For this review, take the finished solid that the model builds, in its own axes (mm). Round coordinates to 2 decimals unless told otherwise and drop trailing zeros. Write each loop counter-clockwise with the first axis right and the second up, starting at its lowest first coordinate (ties: lowest second). Pieces come first, ordered by that corner, then holes.
Autodesk Inventor part; units mm, degrees
ref_plane "YZ Plane" through (0, 0, 0) normal (1, 0, 0) x (0, 1, 0)
ref_plane "XZ Plane" through (0, 0, 0) normal (0, 1, 0) x (-1, 0, 0)
ref_plane "XY Plane" through (0, 0, 0) normal (0, 0, 1) x (1, 0, 0)
sketch "Sketch1" plane through (0, 0, 0) normal (0, 0, 1) x (1, 0, 0)
  circle A0 centre (0, 0) radius 35
  dimension "d0" = 70
extrude "Plate1" add sketch "Sketch1" along normal blind 2
sketch "Sketch2" plane through (0, 0, 0) normal (0, 0, 1) x (1, 0, 0)
  point P0 (0, 0)
  point P1 (28, 0)
  dimension "d2" = 28
hole "Hole1" at (28, 0, 0) direction (0, 0, 1) diameter 6 end through all
pattern_circular "Circular Pattern1" count 3 over 360 about axis through (0, 0, -10) along (0, 0, 1) of "Hole1"
sketch "Sketch3" plane through (0, 0, 2) normal (0, 0, 1) x (1, 0, 0)
  circle A0 centre (0, 0) radius 16.05
  dimension "d13" = 32.1
extrude "Extrusion1" cut sketch "Sketch3" against normal through all
equation "\"d0\" = Внешний_диам_фланца"
equation "\"d8\" = Thickness"
equation "\"d1\" = Thickness"
equation "\"BendRadius\" = Thickness"
equation "\"BendReliefWidth\" = Thickness"
equation "\"BendReliefDepth\" = 0.5 * Thickness"
equation "\"CornerReliefSize\" = 4 * Thickness"
equation "\"MinimumRemnant\" = 2 * Thickness"
equation "\"TransitionRadius\" = BendRadius"
equation "\"JacobiRadiusSize\" = BendRadius"
equation "\"GapSize\" = Thickness"
properties part number "платик крепежный"
(1) We need section D-D, the plane x = -14. Give the boundary of the cut face in (y, z).
Geometry check:
outline: (-32.08, 0) - (-27.25, 0) - (-27.25, 2) - (-32.08, 2) - close; (-21.25, 0) - (-7.85, 0) - (-7.85, 2) - (-21.25, 2) - close; (7.85, 0) - (21.25, 0) - (21.25, 2) - (7.85, 2) - close; (27.25, 0) - (32.08, 0) - (32.08, 2) - (27.25, 2) - close
(2) Mouldability with a two-part tool opening along Y and no side actions: class faces 1 (the face through (30.93, -0.65, 1.01)), 2 (the face through (-12.737, -9.766, 1.014)), 3 (the face through (7, -15, 2)), 4 (the face through (-28, 21, 1)) as pulls with the +Y half, pulls with the -Y half, needs draft (parallel to the pull), parting line crosses it, or undercut.
Geometry check:
face 1: undercut
face 2: undercut
face 3: needs draft
face 4: parting line crosses it
(3) For pin 1 Ø1 at (y, z) = (-21, 0.5) entering from +X; pin 2 Ø5.5 at (x, y) = (-14, 24.25) entering from -Z, all flat-tipped, find the tip position at first contact; note any pin that passes through.
Geometry check:
pin 1: stops at x = 28.37
pin 2: passes through
(4) We need section A-A, the plane x = 0. Give the boundary of the cut face in (y, z).
Geometry check:
outline: (-35, 0) - (-16.05, 0) - (-16.05, 2) - (-35, 2) - close; (16.05, 0) - (35, 0) - (35, 2) - (16.05, 2) - close
(5) We need section B-B, the plane y = 0. Give the boundary of the cut face in (x, z).
Geometry check:
outline: (-35, 0) - (-16.05, 0) - (-16.05, 2) - (-35, 2) - close; (16.05, 0) - (25, 0) - (25, 2) - (16.05, 2) - close; (31, 0) - (35, 0) - (35, 2) - (31, 2) - close
(6) For line 1 along X through (y, z) = (-0.5, 0.1); line 2 along X through (y, z) = (-2, 0.2); line 3 along Y through (x, z) = (-12, 1.45), list the stretches that pass through material, from the lowest coordinate up.
Geometry check:
line 1: x = -35 to -16.04, 16.04 to 25.04, 30.96 to 35
line 2: x = -34.94 to -15.92, 15.92 to 25.76, 30.24 to 34.94
line 3: y = -32.88 to -26.48, -22.01 to -10.66, 10.66 to 22.01, 26.48 to 32.88
(7) We need section C-C, the plane y = 10. Give the boundary of the cut face in (x, z), and give its area (3 significant figures).
Geometry check:
outline: (-33.54, 0) - (-12.55, 0) - (-12.55, 2) - (-33.54, 2) - close; (12.55, 0) - (33.54, 0) - (33.54, 2) - (12.55, 2) - close
area: 83.9 mm2
